CAD build for the part. Positions are in the model's coordinates, mm. Face numbers are marked on the shaded views. Coordinates: 2 decimals unless noted, no trailing zeros. Order: outer loops, then holes, each group sorted by start corner. A loop starts at its lowest first (then second) coordinate and runs counter-clockwise, first axis right, second up. Notation, with made-up numbers: M 22,88 L 37,88 A33 ccw 37,124 Z; hole C 54.25,22.25 d7. An arc over 180 degrees is marked long. Write item = value, one per line.
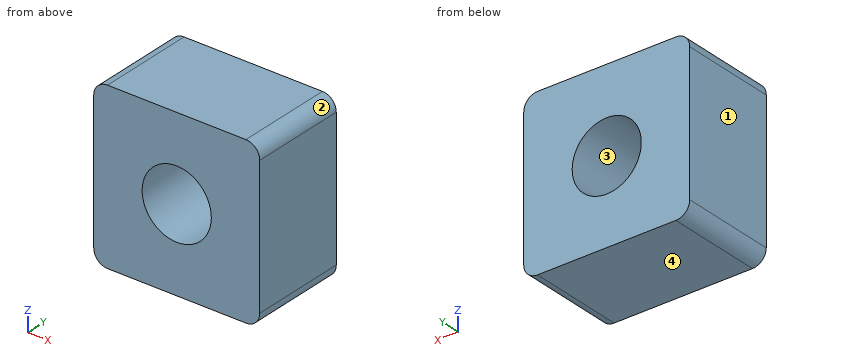
from build123d import *

# Parameters (mm, degrees)
BOSS_EXTRUDE1_DEPTH = 70
SKETCH4_R           = 25
CUT_EXTRUDE4_DEPTH  = 71


with BuildPart() as part:
    # Sketch2 → Boss-Extrude1 (new body)
    with BuildSketch(Plane(origin=(0, 0, 0), x_dir=(1, 0, 0), z_dir=(0, 1, 0))):
        with BuildLine():
            Line((-50, -60), (50, -60))
            ThreePointArc((50, -60), (57.071067812, -57.071067812), (60, -50))
            Line((60, -50), (60, 50))
            ThreePointArc((60, 50), (57.071067812, 57.071067812), (50, 60))
            Line((50, 60), (-50, 60))
            ThreePointArc((-50, 60), (-57.071067812, 57.071067812), (-60, 50))
            Line((-60, 50), (-60, -50))
            ThreePointArc((-60, -50), (-57.071067812, -57.071067812), (-50, -60))
        make_face()
    extrude(amount=BOSS_EXTRUDE1_DEPTH)

    # Sketch4 → Cut-Extrude4 (cut, through all)
    with BuildSketch(Plane.XZ):
        Circle(SKETCH4_R)
    extrude(amount=-CUT_EXTRUDE4_DEPTH, mode=Mode.SUBTRACT)


solid = part.part
(1) Pull direction Z, two halves, no side cores. Call the marked faces 1, 2, 3 and 4: +Z half, -Z half, draft (parallel to the pull), parting line (faces both ways), or undercut.
Evaluation:
face_1 = draft
face_2 = +Z half
face_3 = undercut
face_4 = -Z half
(2) Slice it at C-C, the plane z = 0. Write the cut outline in (x, y), then the cut area to 3 significant figures.
Evaluation:
outline = M -60,0 L -25,0 L -25,70 L -60,70 Z; M 25,0 L 60,0 L 60,70 L 25,70 Z
area = 4,900 mm²
(3) Slice it at B-B, the plane x = 0. Write the cut outline in (y, z), then the cut area to 3 significant figures.
Evaluation:
outline = M 0,-60 L 70,-60 L 70,-25 L 0,-25 Z; M 0,25 L 70,25 L 70,60 L 0,60 Z
area = 4,900 mm²
(4) Slice it at A-A, the plane y = 47. Write the cut outline in (x, z), then the cut area to 3 significant figures.
Evaluation:
outline = M -60,-50 A10 ccw -50,-60 L 50,-60 A10 ccw 60,-50 L 60,50 A10 ccw 50,60 L -50,60 A10 ccw -60,50 Z; hole C 0,0 d50
area = 12,400 mm²
(5) Wall check: line 1 (Z direction, x = 0, y = 30); line 2 (X direction, y = 61.5, z = 8); line 3 (X direction, y = 61, z = 14). Give the ranges that are in metal, low to high. Write a range as from..to.
Evaluation:
line_1 = -60..-25, 25..60
line_2 = -60..-23.69, 23.69..60
line_3 = -60..-20.71, 20.71..60
